Geometry: final body of the model. Coordinates: model frame, mm. A direction names the side the tool comes from. Give positions to 0.01 mm unless a question says otherwise; leave off trailing zeros. Loops run counter-clockwise (first coordinate to the right, second up) from the corner with the lowest first, then second, coordinate; pieces in that order, holes last.
1. Section D-D, the plane x = 9. Output: boundary loops of the cut face in (y, z).
2. Material intervals for line 1 along Y through (x, z) = (32, 1); line 2 along X through (y, z) = (4, 2); line 3 along X through (y, z) = (40, 0.5), sorted ascending.
3. Access query for faces 5 (the face through (60, 43, 3)), 6 (the face through (12, 9.5, 3)). Directions: +Z, -Z, +X, -X, +Y, -Y. A direction counts if a zero-diameter tool reaches every point of the face in a straight line with its end or side. Return the directions, or none.
4. Section A-A, the plane y = 82.5. Output: boundary loops of the cut face in (x, z), then the cut area to 3 significant figures.
5. Draft query along Y for faces 1 (the face through (30, 16.5, 3)), 2 (the face through (16, 64, 0)), 3 (the face through (30, 78, 3)), 4 (the face through (59, 1, 3)). Return one class per face: +Y half, -Y half, draft (parallel to the pull), parting line (faces both ways), or undercut.
6. First-contact query: P1, Ø6, axis at x = 51, y = 61.5, coming from the -Z side. Flat tip, straight axial feed; report the tip coordinate or a pass-through.
7. Section B-B, the plane y = 19.5. Output: boundary loops of the cut face in (x, z).
8. Section C-C, the plane x = 46. Output: boundary loops of the cut face in (y, z).
Autodesk Inventor part; units mm, degrees
ref_plane "YZ Plane" through (0, 0, 0) normal (1, 0, 0) x (0, 1, 0)
ref_plane "XZ Plane" through (0, 0, 0) normal (0, 1, 0) x (-1, 0, 0)
ref_plane "XY Plane" through (0, 0, 0) normal (0, 0, 1) x (1, 0, 0)
sketch "Sketch1" plane through (0, 0, 0) normal (0, 0, 1) x (1, 0, 0)
  line L0 (0, 0) -> (60, 0)
  line L1 (60, 0) -> (60, 87.5)
  line L2 (60, 87.5) -> (0, 87.5)
  line L3 (0, 87.5) -> (0, 0)
  line L4 (54, 30.5589) -> (39.9411, 16.5)
  line L5 (39.9411, 16.5) -> (20.0589, 16.5)
  line L6 (20.0589, 16.5) -> (6, 30.5589)
  line L7 (6, 30.5589) -> (6, 50.4411)
  line L8 (6, 50.4411) -> (20.0589, 64.5)
  line L9 (20.0589, 64.5) -> (39.9411, 64.5)
  line L10 (39.9411, 64.5) -> (54, 50.4411)
  line L11 (54, 50.4411) -> (54, 30.5589)
  line L12 (9, 61.5) -> (51, 61.5) construction
  line L13 (51, 61.5) -> (51, 19.5) construction
  line L14 (51, 19.5) -> (9, 19.5) construction
  line L15 (9, 19.5) -> (9, 61.5) construction
  circle A0 centre (9, 61.5) radius 3.2
  circle A1 centre (9, 19.5) radius 3.2
  circle A2 centre (51, 19.5) radius 3.2
  circle A3 centre (51, 61.5) radius 3.2
  line L16 (8, 9.5) -> (16, 9.5)
  line L17 (16, 9.5) -> (16, 3)
  line L18 (16, 3) -> (8, 3)
  line L19 (8, 3) -> (8, 9.5)
  line L20 (44, 9.5) -> (52, 9.5)
  line L21 (52, 9.5) -> (52, 3)
  line L22 (52, 3) -> (44, 3)
  line L23 (44, 3) -> (44, 9.5)
  line L24 (8, 78) -> (16, 78)
  line L25 (16, 78) -> (16, 71.5)
  line L26 (16, 71.5) -> (8, 71.5)
  line L27 (8, 71.5) -> (8, 78)
  line L28 (44, 78) -> (52, 78)
  line L29 (52, 78) -> (52, 71.5)
  line L30 (52, 71.5) -> (44, 71.5)
  line L31 (44, 71.5) -> (44, 78)
  line L32 (26, 84.5) -> (34, 84.5)
  line L33 (34, 84.5) -> (34, 78)
  line L34 (34, 78) -> (26, 78)
  line L35 (26, 78) -> (26, 84.5)
  line L36 (12, 71.5) -> (12, 9.5) construction
  point P0 (30, 40.5)
  point P1 (30, 61.5)
  point P2 (30, 64.5)
  point P3 (9, 40.5)
  point P4 (6, 40.5)
  point P5 (12, 40.5)
  point P6 (30, 78)
  dimension "d0" = 42
  dimension "d1" = 42
  dimension "d2" = 48
  dimension "d3" = 6.4
  dimension "d4" = 6.4
  dimension "d5" = 6.4
  dimension "d6" = 6.4
  dimension "d7" = 6.5
  dimension "d8" = 8
  dimension "d9" = 6.5
  dimension "d10" = 8
  dimension "d11" = 3
  dimension "d12" = 8
  dimension "d13" = 6.5
  dimension "d14" = 3
  dimension "d15" = 87.5
  dimension "d16" = 6
  dimension "d17" = 6
  dimension "d18" = 8
  dimension "d19" = 8
extrude "Extrusion1" add sketch "Sketch1" along normal blind 6.5
chamfer "Chamfer1" distance 2 angle 45 4 edges at (0, 0, 3.25) (60, 0, 3.25) (60, 87.5, 3.25) (0, 87.5, 3.25)
properties part number "x_iddler_c_mount"
Answers below:
1. outline: (0, 0) - (3, 0) - (3, 6.5) - (0, 6.5) - close; (9.5, 0) - (16.3, 0) - (16.3, 6.5) - (9.5, 6.5) - close; (22.7, 0) - (27.56, 0) - (27.56, 6.5) - (22.7, 6.5) - close; (53.44, 0) - (58.3, 0) - (58.3, 6.5) - (53.44, 6.5) - close; (64.7, 0) - (71.5, 0) - (71.5, 6.5) - (64.7, 6.5) - close; (78, 0) - (87.5, 0) - (87.5, 6.5) - (78, 6.5) - close
2. line 1: y = 0 to 16.5, 64.5 to 78, 84.5 to 87.5
2. line 2: x = 0 to 8, 16 to 44, 52 to 60
2. line 3: x = 0 to 6, 54 to 60
3. face 5: +Z, -Z, +X, +Y, -Y
3. face 6: +Z, -Z
4. outline: (0, 0) - (26, 0) - (26, 6.5) - (0, 6.5) - close; (34, 0) - (60, 0) - (60, 6.5) - (34, 6.5) - close
4. area: 338 mm2
5. face 1: undercut
5. face 2: draft
5. face 3: undercut
5. face 4: -Y half
6. P1: passes through
7. outline: (0, 0) - (5.8, 0) - (5.8, 6.5) - (0, 6.5) - close; (12.2, 0) - (17.06, 0) - (17.06, 6.5) - (12.2, 6.5) - close; (42.94, 0) - (47.8, 0) - (47.8, 6.5) - (42.94, 6.5) - close; (54.2, 0) - (60, 0) - (60, 6.5) - (54.2, 6.5) - close
8. outline: (0, 0) - (3, 0) - (3, 6.5) - (0, 6.5) - close; (9.5, 0) - (22.56, 0) - (22.56, 6.5) - (9.5, 6.5) - close; (58.44, 0) - (71.5, 0) - (71.5, 6.5) - (58.44, 6.5) - close; (78, 0) - (87.5, 0) - (87.5, 6.5) - (78, 6.5) - close
